Source: CAD feature listing. Evaluate the final solid. Frame: model axes, mm. Face numbers are marked on the shaded views. A direction names the side the tool comes from. Give positions to 0.01 mm unless a question says otherwise; leave off trailing zeros. Order: outer loops, then holes, each group sorted by start corner. A loop starts at its lowest first (then second) coordinate and runs counter-clockwise, first axis right, second up.
1) Access query for the marked faces 4, 5 and 6. Directions: +Z, -Z, +X, -X, +Y, -Y. A direction counts if a zero-diameter tool reaches every point of the face in a straight line with its end or side. Return the directions, or none.
2) Section B-B, the plane z = 76.2. Return loops of the section in (x, y).
3) First-contact query: P1, Ø15, axis at y = -15.5, z = 72, coming from the -X side; P2, Ø6, axis at x = -17, z = 22, coming from the -Y side; P3, Ø12, axis at x = -15, z = 59, coming from the +Y side. Flat tips, straight axial feed; report the tip coordinate or a pass-through.
4) Draft query along Z for the marked faces 1, 2 and 3. Return one class per face: released by +Z, released by -Z, zero draft, split by the parting line, or undercut.
5) Material intervals for line 1 (X direction, y = 10, z = 76.2); line 2 (Z direction, x = -9, y = -16.5); line 3 (Y direction, x = -66, z = 50.5), sorted ascending.
6) Section C-C, the plane x = -22. Return loops of the section in (y, z).
7) Section A-A, the plane y = 106.5. Return loops of the section in (x, z).
8) Section D-D, the plane x = 2. Return loops of the section in (y, z), plus the area to 3 significant figures.
```python
from build123d import *

# Parameters (mm, degrees)
F0_W        = 127
F0_H        = 215.9
F1_DEPTH    = 107.95
F2_W        = 50.4830591381
F2_H        = 107.95
F3_DEPTH    = 50.8
F4_W        = 76.2
F4_H        = 44.45
F5_DEPTH    = 76.2
F8_T1_DEPTH = 726.8985851792
F6_R        = 12.7
F9_DEPTH    = 215.901
F7_R        = 12.7
F10_DEPTH   = 127
F11_W       = 25.4
F11_H       = 44.45
F12_DEPTH   = 50.8


# Not quite as in the source:
# - a fillet or chamfer that OpenCascade refuses, or shapes differently, is made with other operations: its cross-section is extruded or revolved along the edge and cut away or added


with BuildPart() as f1:
    # F0 (on Top) → F1 (new body)
    with BuildSketch(Plane.XY):
        with Locations((-16.8368311822, 57.4669408619)):
            Rectangle(F0_W, F0_H)
    extrude(amount=F1_DEPTH)

    # F2 (on face) → F3 (cut)
    with BuildSketch(Plane(origin=(-80.3368311822, 0, 0), x_dir=(0, -1, 0), z_dir=(-1, 0, 0))):
        with Locations((25.241529569, 53.975)):
            Rectangle(F2_W, F2_H)
    extrude(amount=-F3_DEPTH, mode=Mode.SUBTRACT)

    # F4 (on face) → F5 (cut)
    with BuildSketch(Plane.XZ.offset(50.4830591381)):
        with Locations((8.5631688178, 22.225)):
            Rectangle(F4_W, F4_H)
    extrude(amount=-F5_DEPTH, mode=Mode.SUBTRACT)

    # F8: fillet of radius 120.65 on 1 edges, made by hand

    # F8_s2 → F8_t1 (cut)
    with BuildSketch(Plane.YZ.offset(-380.2861237718)):
        with BuildLine():
            ThreePointArc((165.4169408619, 0), (126.1347067484, 76.9902377631), (45.4372238261, 107.95))
            Line((45.4372238261, 107.95), (165.4169408619, 107.95))
            Line((165.4169408619, 107.95), (165.4169408619, 0))
        make_face()
    extrude(amount=F8_T1_DEPTH, mode=Mode.SUBTRACT)

    # F6 (on face) → F9 (cut, through all)
    with BuildSketch(Plane.XZ.offset(50.4830591381)):
        with Locations((8.5631688178, 76.2)):
            Circle(F6_R)
    extrude(amount=-F9_DEPTH, mode=Mode.SUBTRACT)

    # F7 (on face) → F10 (cut)
    with BuildSketch(Plane.YZ.offset(46.6631688178)):
        with Locations((101.9169408619, 44.45)):
            Circle(F7_R)
    extrude(amount=-F10_DEPTH, mode=Mode.SUBTRACT)

    # F11 (on face) → F12 (cut)
    with BuildSketch(Plane(origin=(-80.3368311822, 0, 0), x_dir=(0, -1, 0), z_dir=(-1, 0, 0))):
        with Locations((-12.7, 22.225)):
            Rectangle(F11_W, F11_H)
    extrude(amount=-F12_DEPTH, mode=Mode.SUBTRACT)


solid = f1.part
```
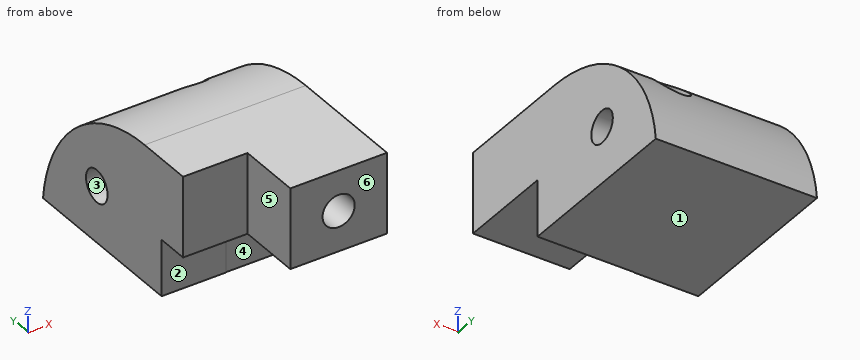
From the geometry:
1. face 4: -Z, +X, -Y
1. face 5: +Z, -Z, -X, -Y
1. face 6: +Z, -Z, +X, -X, -Y
2. outline: (-80.34, 0) - (-29.54, 0) - (-29.54, -50.48) - (-4.14, -50.48) - (-4.14, 127) - (-80.34, 127) - close; (21.26, -50.48) - (46.66, -50.48) - (46.66, 127) - (21.26, 127) - close
3. P1: stops at x = -29.54
3. P2: stops at y = 25.72
3. P3: stops at y = 146.63
4. face 1: released by -Z
4. face 2: zero draft
4. face 3: undercut
5. line 1: x = -80.34 to -4.14, 21.26 to 46.66
5. line 2: z = 44.45 to 107.95
5. line 3: y = 0 to 90.75, 113.08 to 148.21
6. outline: (-50.48, 44.45) - (25.72, 44.45) - (25.72, 0) - (165.42, 0) arc R120.65 ccw to (45.44, 107.95) - (-50.48, 107.95) - close; hole circle Ø25.4 at (101.92, 44.45)
7. outline: (-80.34, 0) - (46.66, 0) - (46.66, 32.61) - (-80.34, 32.61) - close; (-80.34, 56.29) - (46.66, 56.29) - (46.66, 91.36) - (-80.34, 91.36) - close; hole circle Ø25.4 at (8.56, 76.2)
8. outline: (-50.48, 44.45) - (25.72, 44.45) - (25.72, 0) - (165.42, 0) arc R120.65 ccw to (137.46, 65.33) - (-50.48, 65.33) - close; (-50.48, 87.07) - (113.27, 87.07) arc R120.65 ccw to (45.44, 107.95) - (-50.48, 107.95) - close; hole circle Ø25.4 at (101.92, 44.45)
8. area: 12,500 mm2
